Autodesk Inventor part; units mm, degrees
ref_plane "YZ Plane" through (0, 0, 0) normal (1, 0, 0) x (0, 1, 0)
ref_plane "XZ Plane" through (0, 0, 0) normal (0, 1, 0) x (-1, 0, 0)
ref_plane "XY Plane" through (0, 0, 0) normal (0, 0, 1) x (1, 0, 0)
sketch "스케치1" plane through (0, 0, 0) normal (0, 1, 0) x (-1, 0, 0)
  line L0 (0, 0) -> (-30, 0)
  line L1 (-30, 0) -> (-30, -30)
  line L2 (-30, -30) -> (0, -30)
  line L3 (0, -30) -> (0, 0)
  dimension "d0" = 30
  dimension "d1" = 30
extrude "돌출1" add sketch "스케치1" along normal blind 200
sketch "스케치6" plane through (0, 200, 0) normal (0, 1, 0) x (1, 0, 0)
  line L0 (0, 11.85) -> (9.6, 11.85)
  line L1 (9.6, 11.85) -> (9.6, 18.15)
  line L2 (9.6, 18.15) -> (0, 18.15)
  line L3 (0, 18.15) -> (0, 11.85)
  line L4 (0, 30) -> (0, 0)
  line L5 (0, 0) -> (30, 0) construction
  line L6 (15, 0) -> (15, 30) construction
  line L7 (30, 30) -> (0, 30) construction
  line L8 (0, 15) -> (30, 15) construction
  line L9 (11.85, 0) -> (18.15, 0)
  line L10 (18.15, 0) -> (18.15, 9.6)
  line L11 (18.15, 9.6) -> (11.85, 9.6)
  line L12 (11.85, 9.6) -> (11.85, 0)
  line L13 (0, 30) -> (30, 30) construction
  line L14 (11.85, 30) -> (18.15, 30)
  line L15 (18.15, 30) -> (18.15, 20.4)
  line L16 (18.15, 20.4) -> (11.85, 20.4)
  line L17 (11.85, 20.4) -> (11.85, 30)
  line L18 (30, 11.85) -> (20.4, 11.85)
  line L19 (20.4, 11.85) -> (20.4, 18.15)
  line L20 (20.4, 18.15) -> (30, 18.15)
  line L21 (30, 18.15) -> (30, 11.85)
  dimension "d15" = 6.3
  dimension "d16" = 9.6
  dimension "d17" = 9.6
  dimension "d18" = 6.3
extrude "돌출4" cut sketch "스케치6" against normal blind 500
sketch "스케치7" plane through (0, 200, 0) normal (0, 1, 0) x (1, 0, 0)
  circle A0 centre (5.925, 5.925) radius 3
  circle A1 centre (5.925, 24.075) radius 3
  circle A2 centre (24.075, 24.075) radius 3
  circle A3 centre (24.075, 5.925) radius 3
  circle A4 centre (15, 15) radius 2
  line L0 (0, 0) -> (11.85, 0)
  line L1 (0, 11.85) -> (0, 0)
  line L2 (11.85, 30) -> (0, 30)
  line L3 (30, 18.15) -> (30, 30)
  line L4 (9.6, 18.15) -> (9.6, 11.85)
  line L5 (18.15, 20.4) -> (11.85, 20.4)
  point P0 (9.6, 15)
  point P1 (15, 20.4)
  dimension "d21" = 6
  dimension "d22" = 6
  dimension "d23" = 6
  dimension "d24" = 6
  dimension "d25" = 5.925
  dimension "d26" = 5.925
  dimension "d27" = 5.925
  dimension "d28" = 5.925
  dimension "d29" = 4
extrude "돌출5" cut sketch "스케치7" against normal blind 200
properties part number "3030column"
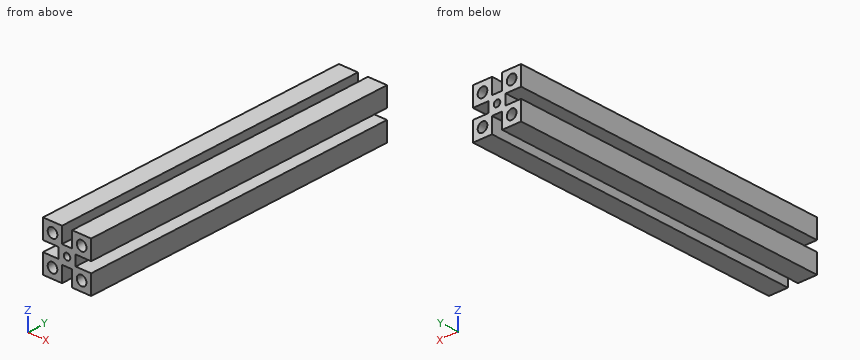
Can you work these out from the model? Positions are in its coordinate system, mm. Give positions to 0.01 mm unless a question says otherwise; leave off trailing zeros. Loops run counter-clockwise (first coordinate to the right, second up) from the corner with the lowest first, then second, coordinate; pieces in that order, holes last. Notation, with made-up numbers: M -21.75,25 L 6.25,25 A24 ccw 6.25,50 Z; hole C 22,-11 d10. An arc over 180 degrees is marked long. Answer in a Markdown table with one row per item.
1. Suppose I cut it at B-B on x = 15. Write out the boundary of the cut face in (y, z), plus the area to 3 significant figures.
Taken from the geometry:
| item | result |
|---|---|
| outline | M 0,-20.4 L 200,-20.4 L 200,-17 L 0,-17 Z; M 0,-13 L 200,-13 L 200,-9.6 L 0,-9.6 Z |
| area | 1,360 mm² |
2. For pin 1 Ø2 at (x, y) = (10, 103) entering from +Z; pin 2 Ø3.5 at (x, z) = (24.075, -24.075) entering from +Y; pin 3 Ø4 at (y, z) = (144.5, -15) entering from +X; pin 4 Ø1.9 at (x, y) = (14, 78) entering from -Z, each with a flat end and sliding along its axis, tell me the tip position at first contact or that it passes through.
Taken from the geometry:
| item | result |
|---|---|
| pin 1 | stops at z = 0 |
| pin 2 | passes through |
| pin 3 | stops at x = 20.4 |
| pin 4 | stops at z = -20.4 |
3. Suppose I cut it at A-A on z = -15. Write out the boundary of the cut face in (x, y), plus the area to 3 significant figures.
Taken from the geometry:
| item | result |
|---|---|
| outline | M 9.6,0 L 13,0 L 13,200 L 9.6,200 Z; M 17,0 L 20.4,0 L 20.4,200 L 17,200 Z |
| area | 1,360 mm² |
4. Suppose I cut it at C-C on y = 137.5. Write out the boundary of the cut face in (x, z) (3 decimals).
Taken from the geometry:
| item | result |
|---|---|
| outline | M 0,-30 L 11.85,-30 L 11.85,-20.4 L 18.15,-20.4 L 18.15,-30 L 30,-30 L 30,-18.15 L 20.4,-18.15 L 20.4,-11.85 L 30,-11.85 L 30,0 L 18.15,0 L 18.15,-9.6 L 11.85,-9.6 L 11.85,0 L 0,0 L 0,-11.85 L 9.6,-11.85 L 9.6,-18.15 L 0,-18.15 Z; hole C 5.925,-24.075 d6; hole C 5.925,-5.925 d6; hole C 15,-15 d4; hole C 24.075,-24.075 d6; hole C 24.075,-5.925 d6 |
5. If I drill on line 1 along Z through (x, y) = (6, 185.5); line 2 along Z through (x, y) = (24.5, 114); line 3 along X through (y, z) = (56, -3.25), over which ranges is the centre line in solid material (lowest first)?
Taken from the geometry:
| item | result |
|---|---|
| line 1 | z = -30 to -27.07, -21.08 to -18.15, -11.85 to -8.92, -2.93 to 0 |
| line 2 | z = -30 to -27.04, -21.11 to -18.15, -11.85 to -8.89, -2.96 to 0 |
| line 3 | x = 0 to 4.57, 7.28 to 11.85, 18.15 to 22.72, 25.43 to 30 |
6. Suppose I cut it at D-D on x = 24.25. Write out the boundary of the cut face in (y, z), plus the area to 3 significant figures.
Taken from the geometry:
| item | result |
|---|---|
| outline | M 0,-30 L 200,-30 L 200,-27.07 L 0,-27.07 Z; M 0,-21.08 L 200,-21.08 L 200,-18.15 L 0,-18.15 Z; M 0,-11.85 L 200,-11.85 L 200,-8.92 L 0,-8.92 Z; M 0,-2.93 L 200,-2.93 L 200,0 L 0,0 Z |
| area | 2,340 mm² |
